Geometry: final body of the model. Coordinates: model frame, mm. Face numbers are marked on the shaded views. A direction names the side the tool comes from. Give positions to 0.01 mm unless a question says otherwise; leave off trailing zeros. Write each loop counter-clockwise with the first axis right and the second up, starting at its lowest first coordinate (ties: lowest second). Pieces come first, ordered by that corner, then holes. Notation, with made-up numbers: M -14.75,80.25 L 28.25,80.25 A23 ccw 28.25,97.25 Z; hole C 44,72 d7. An arc over 180 degrees is marked long. Use a Markdown table: item, result. Add a question column.
1) Section C-C on z = 2.5. Return the cut outline in (x, y) (3 decimals).
2) Pin query (flat end, axial travel): pin 1 (1.5 mm diameter, centred on x = -9.5, y = 27.5, fed in from -Z); pin 2 (1.5 mm diameter, centred on y = -13, z = 1, fed in from +X); pin 3 (2 mm diameter, centred on y = 7.5, z = 2.5, fed in from +X); pin 4 (10 mm diameter, centred on x = -8, y = 9, fed in from +Z). Return the tip coordinate at first contact, or that it passes through.
3) Section D-D on y = 34. Return the cut outline in (x, z).
4) Section A-A on y = 1. Return the cut outline in (x, z), then the cut area to 3 significant figures.
5) Section B-B on x = -16.5. Return the cut outline in (y, z).
6) Draft query along Y for the marked faces 1, 2, 3 and 4. Return one class per face: +Y half, -Y half, draft (parallel to the pull), parting line (faces both ways), or undercut.
7) Set-up query: the marked faces 5 and 6. Return all of +Z, -Z, +X, -X, +Y, -Y with unobstructed straight access to the full face (end or side cutting, diameter ignored); none if empty.
8) Line query: line 1 (X direction, y = 9.5, z = 3.25); line 2 (X direction, y = 17.5, z = 1.75); line 3 (Y direction, x = -6.5, z = 2.75). Output: solid intervals per line, ascending.
```python
from build123d import *

# Parameters (mm, degrees)
CROQUIS1_R              = 40
DISCO_DEPTH             = 5
CORTAR_EXTRUIR1_DEPTH   = 10
CROQUIS7_R              = 5
SALIENTE_EXTRUIR2_DEPTH = 2


with BuildPart() as part:
    # Croquis1 → Disco (new body)
    with BuildSketch(Plane.XY):
        Circle(CROQUIS1_R)
    extrude(amount=DISCO_DEPTH)

    # Croquis6 → Cortar-Extruir1 (cut)
    with BuildSketch(Plane.XY.offset(5)):
        with BuildLine():
            ThreePointArc((20.740877626, 15.325746158), (15.478626449, 5.779368175), (4.761182136, 3.789140187))
            ThreePointArc((4.761182136, 3.789140187), (-7.887176724, 19.835329272), (-28.318599909, 19.700746158))
            ThreePointArc((-28.318599909, 19.700746158), (-30.681508271, 12.662162204), (-23.642924318, 10.299253842))
            ThreePointArc((-23.642924318, 10.299253842), (-12.744392882, 10.515199633), (-5.662082728, 2.228734589))
            ThreePointArc((-5.662082728, 2.228734589), (-13.23431068, -16.748160043), (-2.902046692, -34.375))
            ThreePointArc((-2.902046692, -34.375), (4.375, -32.902046692), (2.902046692, -25.625))
            ThreePointArc((2.902046692, -25.625), (-2.734233567, -16.294567808), (0.900900592, -6.017874775))
            ThreePointArc((0.900900592, -6.017874775), (21.121487404, -3.087169229), (31.220646601, 14.674253842))
            ThreePointArc((31.220646601, 14.674253842), (26.306508271, 20.239884487), (20.740877626, 15.325746158))
        make_face()
    extrude(amount=-CORTAR_EXTRUIR1_DEPTH, mode=Mode.SUBTRACT)

    # Croquis7 → Saliente-Extruir2 (add)
    with BuildSketch(Plane(origin=(0, 0, 0), x_dir=(-1, 0, 0), z_dir=(0, 0, -1))):
        with Locations(Location((0, 30, 0), (0, 0, 180))):
            Circle(CROQUIS7_R)
        with Locations(Location((25.980762114, -15, 0), (0, 0, 180))):
            Circle(CROQUIS7_R)
        with Locations(Location((-25.980762114, -15, 0), (0, 0, 180))):
            Circle(CROQUIS7_R)
    extrude(amount=SALIENTE_EXTRUIR2_DEPTH)


solid = part.part
```
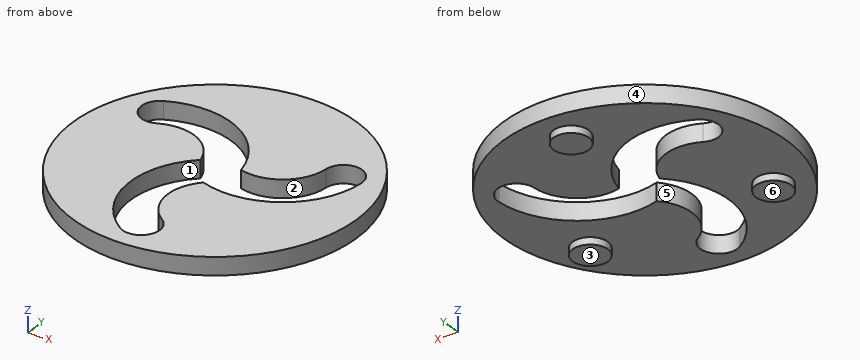
Found:
| question | item | result |
|---|---|---|
| 1 | outline | C 0,0 d80; hole M -28.319,19.701 A5.25 ccw -23.643,10.299 A12.75 cw -5.662,2.229 A23.25 ccw -2.902,-34.375 A5.25 ccw 2.902,-25.625 A12.75 cw 0.901,-6.018 A23.25 ccw 31.221,14.674 A5.25 ccw 20.741,15.326 A12.75 cw 4.761,3.789 A23.25 ccw Z |
| 2 | pin 1 | z = 0 |
| 2 | pin 2 | x = 38.08 |
| 2 | pin 3 | x = 39.47 |
| 2 | pin 4 | z = 5 |
| 3 | outline | M -21.07,0 L -3,0 L -3,-2 L 3,-2 L 3,0 L 21.07,0 L 21.07,5 L -21.07,5 Z |
| 4 | outline | M -39.99,0 L -6.92,0 L -6.92,5 L -39.99,5 Z; M 25.68,0 L 39.99,0 L 39.99,5 L 25.68,5 Z |
| 4 | area | 237 mm² |
| 5 | outline | M -36.44,0 L 11.55,0 L 11.55,5 L -36.44,5 Z; M 22.09,0 L 36.44,0 L 36.44,5 L 22.09,5 Z |
| 6 | face 1 | undercut |
| 6 | face 2 | undercut |
| 6 | face 3 | draft |
| 6 | face 4 | parting line |
| 7 | face 5 | +Z, -Z |
| 7 | face 6 | -Z, +X, -X, +Y, -Y |
| 8 | line 1 | -38.86 to -10.91, 2.72 to 18.91, 30.3 to 38.86 |
| 8 | line 2 | -35.97 to -30.6, -4.04 to 21.36, 30.6 to 35.97 |
| 8 | line 3 | -39.47 to -31.43, 1.43 to 4.46, 19.11 to 39.47 |
